```python
from build123d import *

# Parameters (mm, degrees)
SKETCH1_R           = 1.5
SKETCH1_R_2         = 3.5
BOSS_EXTRUDE1_DEPTH = 3


with BuildPart() as part:
    # Sketch1 → Boss-Extrude1 (new body)
    with BuildSketch(Plane.XY):
        with BuildLine():
            Line((-15, 27.5), (15, 27.5))
            Line((15, 27.5), (15, 30.5))
            Line((15, 30.5), (45, 30.5))
            Line((45, 30.5), (45, 27.5))
            ThreePointArc((45, 27.5), (39.142135624, 13.357864376), (25, 7.5))
            ThreePointArc((25, 7.5), (16.800877501, 4.623903124), (12.195121951, -2.743902439))
            ThreePointArc((12.195121951, -2.743902439), (0, -12.5), (-12.195121951, -2.743902439))
            ThreePointArc((-12.195121951, -2.743902439), (-16.800877501, 4.623903124), (-25, 7.5))
            ThreePointArc((-25, 7.5), (-39.142135624, 13.357864376), (-45, 27.5))
            Line((-45, 27.5), (-45, 30.5))
            Line((-45, 30.5), (-15, 30.5))
            Line((-15, 30.5), (-15, 27.5))
        make_face()
        with Locations((-8.5, 0)):
            Circle(SKETCH1_R, mode=Mode.SUBTRACT)
        with Locations((8.5, 0)):
            Circle(SKETCH1_R, mode=Mode.SUBTRACT)
        Circle(SKETCH1_R_2, mode=Mode.SUBTRACT)
    extrude(amount=BOSS_EXTRUDE1_DEPTH)


solid = part.part
```
Geometry check sheet. Reference: the model listing, model coordinates, mm. A direction names the side the tool comes from. Round coordinates to 2 decimals unless told otherwise and drop trailing zeros. Loops run counter-clockwise (first coordinate to the right, second up) from the corner with the lowest first, then second, coordinate; pieces in that order, holes last. Notation, with made-up numbers: M -14.5,-6 L 10.5,-6 A35 cw 10.5,32 Z; hole C 60,74 d4. An arc over 180 degrees is marked long. Return JSON: item names as keys, results as strings. Group by question number.
(1) Go/stop test with flat-tipped pins: pin 1 (1.5 mm diameter, centred on x = 16.5, z = 2, fed in from -Y); pin 2 (1 mm diameter, centred on y = 21, z = 1.5, fed in from +X). Record where each tip stops, or that it passes through.
(2) Mould release check, pull along Y, two halves, no side actions. Record for faces 1 (the face through (-10, 0, 1)), 2 (the face through (16.9, 4.7, 1.5)), 3 (the face through (1, 14, 3)): pulls with the +Y half, pulls with the -Y half, needs draft (parallel to the pull), parting line crosses it, or undercut.
(3) Section check B-B, the plane z = 2.1. Enter the section's corners in (x, y) (3 decimals), and give its area (3 significant figures).
(4) Scan lines: line 1 along Y through (x, z) = (-8.5, 2.3); line 2 along X through (y, z) = (-3, 1.45); line 3 along Y through (x, z) = (-9.5, 1.35). Record each from-to range of solid material in increasing order. Write a range as [from, to].
(5) Section check C-C, the plane y = 0. Enter the section's corners in (x, z), and give its area (3 significant figures).
(6) Set-up check for faces 4 (the face through (-15, 29, 1)), 5 (the face through (3.233, -1.341, 1.479)): record each of +Z, -Z, +X, -X, +Y, -Y from which the full face is reachable in a straight line by a thin tool's end or side.
(7) Section check A-A, the plane x = 0. Enter the section's corners in (y, z).
(8) Section check D-D, the plane x = -26.5. Enter the section's corners in (y, z).
Data:
{
 "1": {"pin 1": "y = 3.69", "pin 2": "x = 44.08"},
 "2": {"face 1": "undercut", "face 2": "pulls with the -Y half", "face 3": "needs draft"},
 "3": {"outline": "M -45,27.5 A20 ccw -25,7.5 A13.125 cw -12.195,-2.744 A12.5 ccw 12.195,-2.744 A13.125 cw 25,7.5 A20 ccw 45,27.5 L 45,30.5 L 15,30.5 L 15,27.5 L -15,27.5 L -15,30.5 L -45,30.5 Z; hole C -8.5,0 d3; hole C 0,0 d7; hole C 8.5,0 d3", "area": "2,250 mm²"},
 "4": {"line 1": "[-9.17, -1.5], [1.5, 27.5]", "line 2": "[-12.13, -1.8], [1.8, 12.13]", "line 3": "[-8.12, -1.12], [1.12, 27.5]"},
 "5": {"outline": "M -13.14,0 L -10,0 L -10,3 L -13.14,3 Z; M -7,0 L -3.5,0 L -3.5,3 L -7,3 Z; M 3.5,0 L 7,0 L 7,3 L 3.5,3 Z; M 10,0 L 13.14,0 L 13.14,3 L 10,3 Z", "area": "39.8 mm²"},
 "6": {"face 4": "+Z, -Z, +Y", "face 5": "+Z, -Z"},
 "7": {"outline": "M -12.5,0 L -3.5,0 L -3.5,3 L -12.5,3 Z; M 3.5,0 L 27.5,0 L 27.5,3 L 3.5,3 Z"},
 "8": {"outline": "M 7.56,0 L 30.5,0 L 30.5,3 L 7.56,3 Z"}
}
